Verification items for the finished model (mm, model axes). Face numbers are marked on the shaded views. A direction names the side the tool comes from. Coordinates: 2 decimals unless noted, no trailing zeros. Loops run counter-clockwise (first coordinate to the right, second up) from the corner with the lowest first, then second, coordinate; pieces in that order, holes last. Notation, with made-up numbers: (29.5, 3.25) -> (45.5, 3.25) arc R22 cw to (45.5, 28.25) -> close; hole circle Ø9 at (-36, 73). An arc over 180 degrees is marked (long way). Answer as a JSON object with one key per item and string values. Group by question number.
Q1. Scan lines: L1, parallel to Z at x = 0, y = 7 (3 decimals); L2, parallel to Z at x = 29.5, y = 10.25; L3, parallel to Y at x = -4, z = -22. Record each from-to range of solid material in increasing order.
Q2. Gauge pin test, flat ends, axial feed: pin 1 Ø2 at (y, z) = (3, 4) entering from +X; pin 2 Ø1 at (y, z) = (6, 7) entering from -X; pin 3 Ø5.5 at (x, z) = (36, 12) entering from +Y. Record the tip position at first contact, or that the pin passes through.
Q3. Cross-section at C-C on y = 1. Record the boundary of the cut face in (x, z) (3 decimals), and give its area (3 significant figures).
Q4. Release check for a two-part mould opening along Z. For the marked faces 1, 2, 3 and 4 record: released by +Z, released by -Z, zero draft, split by the parting line, or undercut.
Q5. Cross-section at D-D on z = -12.5. Record the boundary of the cut face in (x, y), and give its area (3 significant figures).
Q6. Cross-section at A-A on z = 0. Record the boundary of the cut face in (x, y) (3 decimals).
Q7. Set-up check for the marked faces 5, 6 and 7: record each of +Z, -Z, +X, -X, +Y, -Y from which the full face is reachable in a straight line by a thin tool's end or side.
Q8. Cross-section at B-B on x = 0. Record the boundary of the cut face in (y, z) (3 decimals).
```python
from build123d import *

# Parameters (mm, degrees)
SKETCH1_R           = 41.275
BOSS_EXTRUDE1_DEPTH = 12.7
SKETCH1_4_R         = 2.15
SKETCH1_4_R_2       = 1.905
CUT_EXTRUDE2_DEPTH  = 60.737268518
SKETCH1_5_R         = 7.62
SKETCH1_5_R_2       = 1.905
CUT_EXTRUDE3_DEPTH  = 5.08
CUT_EXTRUDE4_START  = 5.08
SKETCH1_6_R         = 2.15
CUT_EXTRUDE4_DEPTH  = 7.62
FILLET1_R           = 5.08


with BuildPart() as part:
    # Sketch1 → Boss-Extrude1 (new body)
    with BuildSketch(Plane(origin=(0, 0, 0), x_dir=(1, 0, 0), z_dir=(0, 1, 0))):
        with Locations(Location((0, 0, 0), (0, 0, 270))):
            Circle(SKETCH1_R)
    extrude(amount=BOSS_EXTRUDE1_DEPTH)

    # Sketch1<4> → Cut-Extrude2 (cut, through all)
    with BuildSketch(Plane(origin=(0, 0, 0), x_dir=(1, 0, 0), z_dir=(0, 1, 0))):
        with Locations(Location((-34.925, 0, 0), (0, 0, 270))):
            Circle(SKETCH1_4_R)
        with Locations(Location((34.925, 0, 0), (0, 0, 270))):
            Circle(SKETCH1_4_R)
        with Locations(Location((0, 23.876, 0), (0, 0, 270))):
            Circle(SKETCH1_4_R_2)
        with Locations(Location((0, -23.876, 0), (0, 0, 270))):
            Circle(SKETCH1_4_R_2)
    extrude(amount=CUT_EXTRUDE2_DEPTH, mode=Mode.SUBTRACT)

    # Sketch1<5> → Cut-Extrude3 (cut)
    # profile 1 of 2: a face of its own
    with BuildSketch(Plane(origin=(0, 0, 0), x_dir=(1, 0, 0), z_dir=(0, 1, 0))):
        with Locations(Location((0, -23.876, 0), (0, 0, 270))):
            Circle(SKETCH1_5_R)
        with Locations(Location((0, -23.876, 0), (0, 0, 270))):
            Circle(SKETCH1_5_R_2, mode=Mode.SUBTRACT)
    # profile 2 of 2: a face of its own
    with BuildSketch(Plane(origin=(0, 0, 0), x_dir=(1, 0, 0), z_dir=(0, 1, 0))):
        with Locations(Location((0, 23.876, 0), (0, 0, 270))):
            Circle(SKETCH1_5_R)
        with Locations(Location((0, 23.876, 0), (0, 0, 270))):
            Circle(SKETCH1_5_R_2, mode=Mode.SUBTRACT)
    extrude(amount=CUT_EXTRUDE3_DEPTH, mode=Mode.SUBTRACT)

    # Sketch1<6> → Cut-Extrude4 (cut)
    # profile 1 of 2: a face of its own
    with BuildSketch(Plane(origin=(0, 0, 0), x_dir=(1, 0, 0), z_dir=(0, 1, 0)).offset(CUT_EXTRUDE4_START)):
        with BuildLine():
            ThreePointArc((-35.017363636, 21.849710958), (-41.275, 0), (-35.017363636, -21.849710958))
            Line((-35.017363636, -21.849710958), (-24.621881181, -7.425344611))
            ThreePointArc((-24.621881181, -7.425344611), (-22.225, 0), (-24.621881181, 7.425344611))
            Line((-24.621881181, 7.425344611), (-35.017363636, 21.849710958))
        make_face()
        with Locations(Location((-34.925, 0, 0), (0, 0, 270))):
            Circle(SKETCH1_6_R, mode=Mode.SUBTRACT)
    # profile 2 of 2: a face of its own
    with BuildSketch(Plane(origin=(0, 0, 0), x_dir=(1, 0, 0), z_dir=(0, 1, 0)).offset(CUT_EXTRUDE4_START)):
        with BuildLine():
            Line((35.017363636, 21.849710958), (24.621881181, 7.425344611))
            ThreePointArc((24.621881181, 7.425344611), (22.225, 0), (24.621881181, -7.425344611))
            Line((24.621881181, -7.425344611), (35.017363636, -21.849710958))
            ThreePointArc((35.017363636, -21.849710958), (41.275, 0), (35.017363636, 21.849710958))
        make_face()
        with Locations(Location((34.925, 0, 0), (0, 0, 270))):
            Circle(SKETCH1_6_R, mode=Mode.SUBTRACT)
    extrude(amount=CUT_EXTRUDE4_DEPTH, mode=Mode.SUBTRACT)

    # Fillet1
    fillet1_edges = [part.edges().sort_by_distance(p)[0] for p in [
        (35.017363636, 8.89, -21.849710958),
        (35.017363636, 8.89, 21.849710958),
        (-35.017363636, 8.89, 21.849710958),
        (-35.017363636, 8.89, -21.849710958),
    ]]
    fillet(fillet1_edges, radius=FILLET1_R)


solid = part.part
```
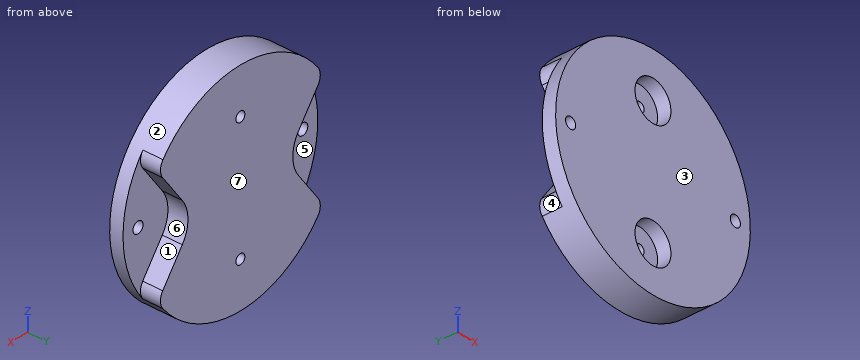
Computed values:
{
 "1": {"L1": "z = -41.275 to -25.781, -21.971 to 21.971, 25.781 to 41.275", "L2": "z = -28.87 to -14.19, 14.19 to 28.87", "L3": "y = 5.08 to 12.7"},
 "2": {"pin 1": "stops at x = 41.17", "pin 2": "stops at x = -24.68", "pin 3": "stops at y = 5.08"},
 "3": {"outline": "circle Ø82.55 at (0, 0); hole circle Ø4.3 at (-34.925, 0); hole circle Ø15.24 at (0, -23.876); hole circle Ø15.24 at (0, 23.876); hole circle Ø4.3 at (34.925, 0)", "area": "4,960 mm²"},
 "4": {"face 1": "undercut", "face 2": "split by the parting line", "face 3": "zero draft", "face 4": "undercut"},
 "5": {"outline": "(-39.34, 0) -> (39.34, 0) -> (39.34, 5.08) -> (28.28, 5.08) -> (28.28, 12.7) -> (-28.28, 12.7) -> (-28.28, 5.08) -> (-39.34, 5.08) -> close", "area": "831 mm²"},
 "6": {"outline": "(-41.275, 0) -> (-37.075, 0) -> (-37.075, 5.08) -> (-41.275, 5.08) -> close; (-32.775, 0) -> (32.775, 0) -> (32.775, 5.08) -> (22.225, 5.08) -> (22.225, 12.7) -> (-22.225, 12.7) -> (-22.225, 5.08) -> (-32.775, 5.08) -> close; (37.075, 0) -> (41.275, 0) -> (41.275, 5.08) -> (37.075, 5.08) -> close"},
 "7": {"face 5": "-X, +Y", "face 6": "+X, +Y", "face 7": "+Z, -Z, +X, -X, +Y"},
 "8": {"outline": "(0, -41.275) -> (12.7, -41.275) -> (12.7, -25.781) -> (5.08, -25.781) -> (5.08, -31.496) -> (0, -31.496) -> close; (0, -16.256) -> (5.08, -16.256) -> (5.08, -21.971) -> (12.7, -21.971) -> (12.7, 21.971) -> (5.08, 21.971) -> (5.08, 16.256) -> (0, 16.256) -> close; (0, 31.496) -> (5.08, 31.496) -> (5.08, 25.781) -> (12.7, 25.781) -> (12.7, 41.275) -> (0, 41.275) -> close"}
}
